For this review, use the dimensioned drawing (mm, ordinates from the lowest corner) and the shaded views. Coordinates: 2 decimals unless noted, no trailing zeros. Loops run counter-clockwise (first coordinate to the right, second up) from the corner with the lowest first, then second, coordinate; pieces in that order, holes last. Notation, with made-up numbers: (68, 54) -> (111, 54) arc R6 ccw to (111, 65) -> close; hole circle Ø4 at (54, -1.75). An arc over 180 degrees is marked (long way). Answer as a JSON object with one key per item and string values.
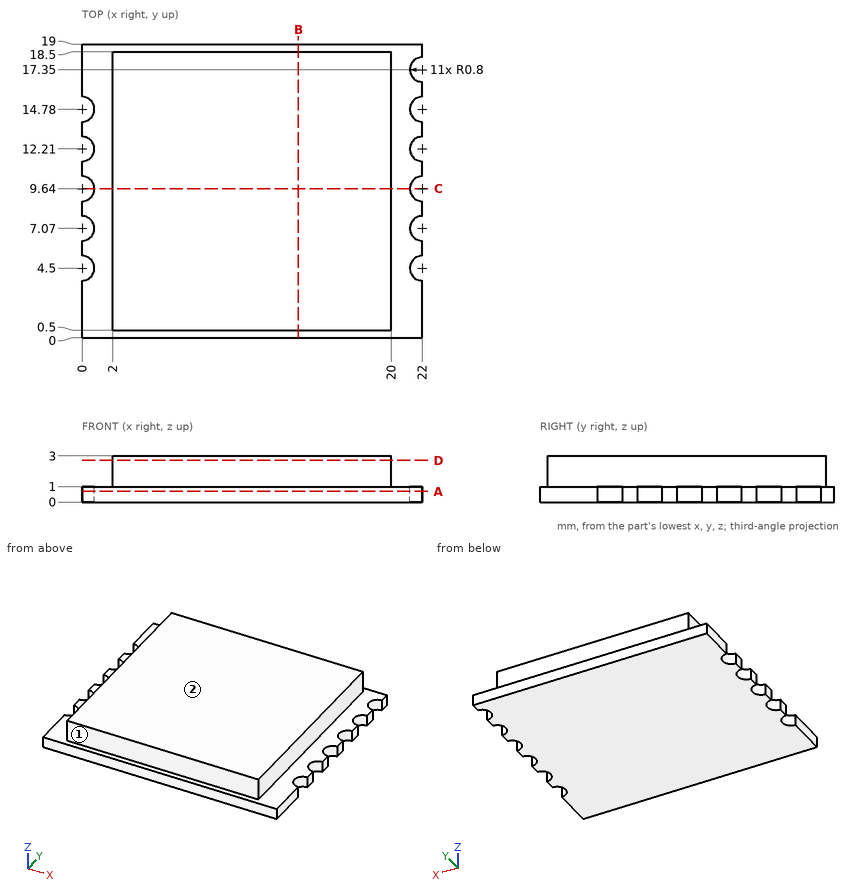
1) Add section C-C, the plane y = 9.64. Give the boundary of the cut face in (x, z).
Completed:
{"outline": "(0.8, 0) -> (21.2, 0) -> (21.2, 1) -> (20, 1) -> (20, 3) -> (2, 3) -> (2, 1) -> (0.8, 1) -> close"}
2) Add section A-A, the plane z = 0.7. Give the boundary of the cut face in (x, y), and give its area (3 significant figures).
Completed:
{"outline": "(0, 0) -> (22, 0) -> (22, 3.7) arc R0.8 cw to (22, 5.3) -> (22, 6.27) arc R0.8 cw to (22, 7.87) -> (22, 8.84) arc R0.8 cw to (22, 10.44) -> (22, 11.41) arc R0.8 cw to (22, 13.01) -> (22, 13.98) arc R0.8 cw to (22, 15.58) -> (22, 16.55) arc R0.8 cw to (22, 18.15) -> (22, 19) -> (0, 19) -> (0, 15.58) arc R0.8 cw to (0, 13.98) -> (0, 13.01) arc R0.8 cw to (0, 11.41) -> (0, 10.44) arc R0.8 cw to (0, 8.84) -> (0, 7.87) arc R0.8 cw to (0, 6.27) -> (0, 5.3) arc R0.8 cw to (0, 3.7) -> close", "area": "407 mm²"}
3) Add section B-B, the plane x = 14. Give the boundary of the cut face in (y, z).
Completed:
{"outline": "(0, 0) -> (19, 0) -> (19, 1) -> (18.5, 1) -> (18.5, 3) -> (0.5, 3) -> (0.5, 1) -> (0, 1) -> close"}
4) Wall thickness on probe 1 along Y at (x, z) = (18.5, 1.65); probe 2 along X at (y, z) = (12.25, 1.55); probe 3 along Z at (x, y) = (20.5, 9.5): over which ranges is each line inside the solid? List them lowest first.
Completed:
{"probe 1": "0.5 to 18.5", "probe 2": "2 to 20", "probe 3": "0 to 1"}
5) Add section D-D, the plane z = 2.7. Give the boundary of the cut face in (x, y), and give its area (3 significant figures).
Completed:
{"outline": "(2, 0.5) -> (20, 0.5) -> (20, 18.5) -> (2, 18.5) -> close", "area": "324 mm²"}
6) Clearance check with flat-ended pins moving along their axes: pin 1 Ø1.6 at (y, z) = (7, 2.5) entering from +X; pin 2 Ø0.6 at (x, z) = (8.5, 2) entering from +Y; pin 3 Ø1 at (x, z) = (8, 2) entering from -Y; pin 4 Ø3 at (x, y) = (8, 11) entering from -Z. State where each tip first meets the part, or that it passes through.
Completed:
{"pin 1": "x = 20", "pin 2": "y = 18.5", "pin 3": "y = 0.5", "pin 4": "z = 0"}
7) The part is to be moulded in two halves that separate along Y. For the marked faces 1 and 2, say which applies: pulls with the +Y half, pulls with the -Y half, needs draft (parallel to the pull), parting line crosses it, or undercut.
Completed:
{"face 1": "pulls with the -Y half", "face 2": "needs draft"}
